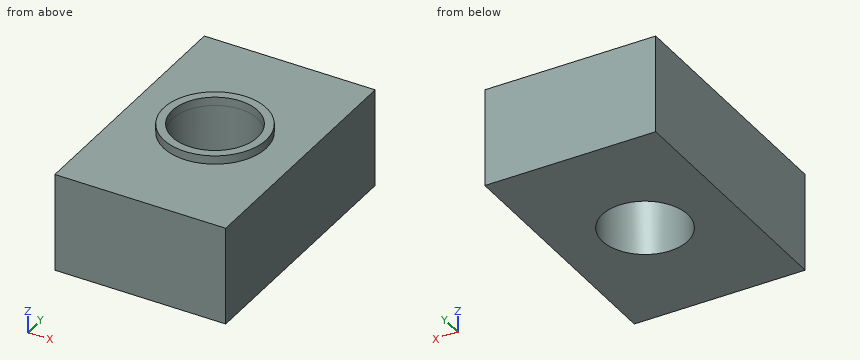
from build123d import *

# Parameters (mm, degrees)
F0_W     = 80
F0_H     = 120
F1_DEPTH = 46
F2_R     = 20
F3_DEPTH = 65
F2_R_2   = 24
F4_DEPTH = 4


with BuildPart() as f1:
    # F0 (on Top) → F1 (new body)
    with BuildSketch(Plane.XY):
        Rectangle(F0_W, F0_H)
    extrude(amount=F1_DEPTH)

    # F2 (on face) → F3 (cut)
    with BuildSketch(Plane.XY.offset(46)):
        Circle(F2_R)
    extrude(amount=-F3_DEPTH, mode=Mode.SUBTRACT)

    # F2 (on face) → F4 (join)
    with BuildSketch(Plane.XY.offset(46)):
        Circle(F2_R_2)
        Circle(F2_R, mode=Mode.SUBTRACT)
    extrude(amount=F4_DEPTH)


solid = f1.part
Geometry: final body of the model. Coordinates: model frame, mm. Give positions to 0.01 mm unless a question says otherwise; leave off trailing zeros. Write each loop counter-clockwise with the first axis right and the second up, starting at its lowest first coordinate (ties: lowest second). Pieces come first, ordered by that corner, then holes. Notation, with made-up numbers: (85, -14) -> (129, -14) arc R16 cw to (129, 9) -> close; hole circle Ø2 at (-20, 41.5). An arc over 180 degrees is marked (long way). Answer as a JSON object with one key per item and string values.
1. Ray query, probe 1 along Y at (x, z) = (0, 48); probe 2 along Y at (x, z) = (0, 22); probe 3 along Z at (x, y) = (10.5, -45). Return the intervals inside material, ascending. Write a range as from..to.
Ans:
{"probe 1": "y = -24..-20, 20..24", "probe 2": "y = -60..-20, 20..60", "probe 3": "z = 0..46"}
2. Cut plane D-D on y = -41. Output: boundary loops of the cut face in (x, z), and give its area (3 significant figures).
Ans:
{"outline": "(-40, 0) -> (40, 0) -> (40, 46) -> (-40, 46) -> close", "area": "3,680 mm^2"}
3. Cut plane B-B on y = 0. Output: boundary loops of the cut face in (x, z).
Ans:
{"outline": "(-40, 0) -> (-20, 0) -> (-20, 50) -> (-24, 50) -> (-24, 46) -> (-40, 46) -> close; (20, 0) -> (40, 0) -> (40, 46) -> (24, 46) -> (24, 50) -> (20, 50) -> close"}
4. Cut plane A-A on x = 0. Output: boundary loops of the cut face in (y, z), and give its area (3 significant figures).
Ans:
{"outline": "(-60, 0) -> (-20, 0) -> (-20, 50) -> (-24, 50) -> (-24, 46) -> (-60, 46) -> close; (20, 0) -> (60, 0) -> (60, 46) -> (24, 46) -> (24, 50) -> (20, 50) -> close", "area": "3,710 mm^2"}
5. Contact query for flat-ended pins moving along their axis: pin 1 (24 mm diameter, centred on x = 0, y = 0, fed in from +Z); pin 2 (8 mm diameter, centred on x = 27.5, y = 4.5, fed in from -Z); pin 3 (3 mm diameter, centred on x = -15, y = -24.5, fed in from +Z). Output: stop coordinate, or through.
Ans:
{"pin 1": "passes through", "pin 2": "stops at z = 0", "pin 3": "stops at z = 46"}
6. Cut plane C-C on z = 18.5. Output: boundary loops of the cut face in (x, y), and give its area (3 significant figures).
Ans:
{"outline": "(-40, -60) -> (40, -60) -> (40, 60) -> (-40, 60) -> close; hole circle Ø40 at (0, 0)", "area": "8,340 mm^2"}
